Work out the finished part from the listing and answer in its coordinate system (mm). A direction names the side the tool comes from. Round coordinates to 2 decimals unless told otherwise and drop trailing zeros. Loops run counter-clockwise (first coordinate to the right, second up) from the corner with the lowest first, then second, coordinate; pieces in that order, holes last.
from build123d import *

# Parameters (mm, degrees)
F0_R     = 9.525
F1_DEPTH = 25.4
F3_DEPTH = 25.401
F4_DEPTH = 11.0998
F6_DEPTH = 9.525


with BuildPart() as f1:
    # F0 (on Front) → F1 (new body)
    with BuildSketch(Plane.XZ):
        Circle(F0_R)
    extrude(amount=F1_DEPTH)

    # F2 (on face) → F3 (cut, through all)
    with BuildSketch(Plane.XZ.offset(25.4)):
        with BuildLine():
            ThreePointArc((-4.7625, 0), (-3.367596, -3.367596), (0, -4.7625))
            ThreePointArc((0, -4.7625), (3.367596, -3.367596), (4.7625, 0))
            ThreePointArc((4.7625, 0), (3.367596, 3.367596), (0, 4.7625))
            ThreePointArc((0, 4.7625), (-3.367596, 3.367596), (-4.7625, 0))
        make_face()
    extrude(amount=-F3_DEPTH, mode=Mode.SUBTRACT)

    # F2 (on face) → F4 (cut)
    with BuildSketch(Plane.XZ.offset(25.4)):
        with BuildLine():
            Line((0, -4.7625), (4.7625, -4.7625))
            Line((4.7625, -4.7625), (4.7625, 0))
            ThreePointArc((4.7625, 0), (3.367596, -3.367596), (0, -4.7625))
        make_face()
        with BuildLine():
            Line((-4.7625, -4.7625), (0, -4.7625))
            ThreePointArc((0, -4.7625), (-3.367596, -3.367596), (-4.7625, 0))
            Line((-4.7625, 0), (-4.7625, -4.7625))
        make_face()
        with BuildLine():
            ThreePointArc((0, 4.7625), (3.367596, 3.367596), (4.7625, 0))
            Line((4.7625, 0), (4.7625, 4.7625))
            Line((4.7625, 4.7625), (0, 4.7625))
        make_face()
        with BuildLine():
            Line((-4.7625, 4.7625), (-4.7625, 0))
            ThreePointArc((-4.7625, 0), (-3.367596, 3.367596), (0, 4.7625))
            Line((0, 4.7625), (-4.7625, 4.7625))
        make_face()
    extrude(amount=-F4_DEPTH, mode=Mode.SUBTRACT)

    # F5 (on face) → F6 (cut)
    with BuildSketch(Plane(origin=(0, 0, 0), x_dir=(-1, 0, 0), z_dir=(0, 1, 0))):
        Polygon((7.3025, -0.000211), (3.651432, 6.324045), (-3.651068, 6.324256), (-7.3025, 0.000211), (-3.651432, -6.324045), (3.651068, -6.324256), align=None)
    extrude(amount=-F6_DEPTH, mode=Mode.SUBTRACT)


solid = f1.part
Item 1: Each of these flat-tipped pins is pushed along its axis until it touches: P1, Ø1, axis at x = -5, y = -10, coming from the +Z side (3 decimals); P2, Ø2, axis at x = -1.5, y = -4.5, coming from the -Z side; P3, Ø6.5, axis at x = -1, z = 1.5, coming from the +Y side (3 decimals). Where does it stop, or does it pass through?
Item 2: For faces 1 (the face through (0, -25.4, -6)), 2 (the face through (0, -20, 4.762)), 3 (the face through (-5, -9.525, 0)), determine the directions among +Z, -Z, +X, -X, +Y, -Y from which every point of the face is accessible in a straight line to the end or side of a thin tool.
Item 3: Determine the mould class of faces 4 (the face through (-7.559, -12.522, -5.796)), 5 (the face through (4, -14.3, -4)), 6 (the face through (6.2, 0, 2.3)) for opening direction Z: pulls with the +Z half, pulls with the -Z half, needs draft (parallel to the pull), parting line crosses it, or undercut.
Item 4: Section C-C, the plane x = -2 is taken. Give the vertices of the cut face in (y, z) (1 decimal), plus the area to 3 significant figures.
Item 5: Straight lines are drawn through the part: line 1 (Z direction, x = -2, y = -20.5); line 2 (X direction, y = -16, z = 0.5); line 3 (X direction, y = -3.25, z = 5). For each, find the intervals that lie inside material, in ascending order.
Item 6: Section D-D, the plane x = 6.75 is taken. Give the vertices of the cut face in (y, z) (3 decimals).
Answer below:
1. P1: stops at z = 8.395
1. P2: stops at z = -9.51
1. P3: stops at y = -9.525
2. face 1: +Z, -Z, +X, -X, -Y
2. face 2: -Y
2. face 3: +Y
3. face 4: parting line crosses it
3. face 5: undercut
3. face 6: needs draft
4. outline: (-25.4, -9.3) - (0, -9.3) - (0, -6.3) - (-9.5, -6.3) - (-9.5, -4.3) - (-14.3, -4.3) - (-14.3, -4.8) - (-25.4, -4.8) - close; (-25.4, 4.8) - (-14.3, 4.8) - (-14.3, 4.3) - (-9.5, 4.3) - (-9.5, 6.3) - (0, 6.3) - (0, 9.3) - (-25.4, 9.3) - close
4. area: 206 mm2
5. line 1: z = -9.31 to -4.76, 4.76 to 9.31
5. line 2: x = -9.51 to -4.76, 4.76 to 9.51
5. line 3: x = -8.11 to -4.42, 4.42 to 8.11
6. outline: (-25.4, -6.72) - (0, -6.72) - (0, -0.957) - (-9.525, -0.957) - (-9.525, 0.957) - (0, 0.957) - (0, 6.72) - (-25.4, 6.72) - close
